```python
from build123d import *

# Parameters (mm, degrees)
SKETCH1_W           = 481.5
SKETCH1_H           = 721.5
BOSS_EXTRUDE1_DEPTH = 100
SHELL1_T            = -0.75
SKETCH2_R           = 13.5
CUT_EXTRUDE1_DEPTH  = 10


with BuildPart() as part:
    # Sketch1 → Boss-Extrude1 (new body)
    with BuildSketch(Plane(origin=(0, 0, 0), x_dir=(1, 0, 0), z_dir=(0, 1, 0))):
        Rectangle(SKETCH1_W, SKETCH1_H)
    extrude(amount=BOSS_EXTRUDE1_DEPTH)

    # Shell1
    shell1_openings = [part.faces().sort_by_distance(p)[0] for p in [
        (0, 100, 0),
    ]]
    offset(amount=SHELL1_T, openings=shell1_openings, kind=Kind.INTERSECTION)

    # Sketch2 → Cut-Extrude1 (cut)
    with BuildSketch(Plane(origin=(0, 0.75, 0), x_dir=(1, 0, 0), z_dir=(0, 1, 0))):
        with Locations((120.75, -310.75)):
            Circle(SKETCH2_R)
    extrude(amount=-CUT_EXTRUDE1_DEPTH, mode=Mode.SUBTRACT)


solid = part.part
```
Geometry check sheet. Reference: the model listing, model coordinates, mm. A direction names the side the tool comes from. Round coordinates to 2 decimals unless told otherwise and drop trailing zeros. Write each loop counter-clockwise with the first axis right and the second up, starting at its lowest first coordinate (ties: lowest second). Pieces come first, ordered by that corner, then holes. Notation, with made-up numbers: (71.25, -28) -> (78.25, -28) arc R23 ccw to (78.25, 11) -> close; hole circle Ø9 at (57, -29). An arc over 180 degrees is marked (long way). Put each result on its own line as item: value.
1) Access from +Z, -Z, +X, -X, +Y, -Y to the whole of each face (thin tool, end or side, straight path). Record for faces 4 (the face through (-3, 49, 360.75)), 5 (the face through (-3, 0.75, -5)).
Recorded:
face 4: +Z, +X, -X, +Y, -Y
face 5: +Y
2) Release check for a two-part mould opening along X. For faces 1 (the face through (240.75, 49, 5)), 2 (the face through (-3, 0, -5)), 3 (the face through (-240, 50, 5)) record: pulls with the +X half, pulls with the -X half, needs draft (parallel to the pull), parting line crosses it, or undercut.
Recorded:
face 1: pulls with the +X half
face 2: needs draft
face 3: undercut
3) Cross-section at D-D, the plane x = -87. Enter the section's corners in (y, z).
Recorded:
outline: (0, -360.75) -> (100, -360.75) -> (100, -360) -> (0.75, -360) -> (0.75, 360) -> (100, 360) -> (100, 360.75) -> (0, 360.75) -> close
4) Depth check by flat-ended pin: P1, Ø10, axis at x = 33, z = -49, coming from the +Y side. Enter the tip coordinate at first touch or a pass-through.
Recorded:
P1: stops at y = 0.75
5) Thickness scan on probe 1 along Z at (x, y) = (120.75, 0.55); probe 2 along X at (y, z) = (86, 84.5); probe 3 along Z at (x, y) = (-183, 52). Record the ranges inside material, lowest first. Write a range as from..to.
Recorded:
probe 1: z = -360.75..297.25, 324.25..360.75
probe 2: x = -240.75..-240, 240..240.75
probe 3: z = -360.75..-360, 360..360.75
6) Cross-section at A-A, the plane z = 310.75. Enter the section's corners in (x, y), plus the area to 3 significant figures.
Recorded:
outline: (-240.75, 0) -> (107.25, 0) -> (107.25, 0.75) -> (-240, 0.75) -> (-240, 100) -> (-240.75, 100) -> close; (134.25, 0) -> (240.75, 0) -> (240.75, 100) -> (240, 100) -> (240, 0.75) -> (134.25, 0.75) -> close
area: 490 mm2
7) Cross-section at B-B, the plane x = 120.75. Enter the section's corners in (y, z), plus the area to 3 significant figures.
Recorded:
outline: (0, -360.75) -> (100, -360.75) -> (100, -360) -> (0.75, -360) -> (0.75, 297.25) -> (0, 297.25) -> close; (0, 324.25) -> (0.75, 324.25) -> (0.75, 360) -> (100, 360) -> (100, 360.75) -> (0, 360.75) -> close
area: 670 mm2
8) Cross-section at C-C, the plane y = 25. Enter the section's corners in (x, z).
Recorded:
outline: (-240.75, -360.75) -> (240.75, -360.75) -> (240.75, 360.75) -> (-240.75, 360.75) -> close; hole (-240, -360) -> (240, -360) -> (240, 360) -> (-240, 360) -> close
